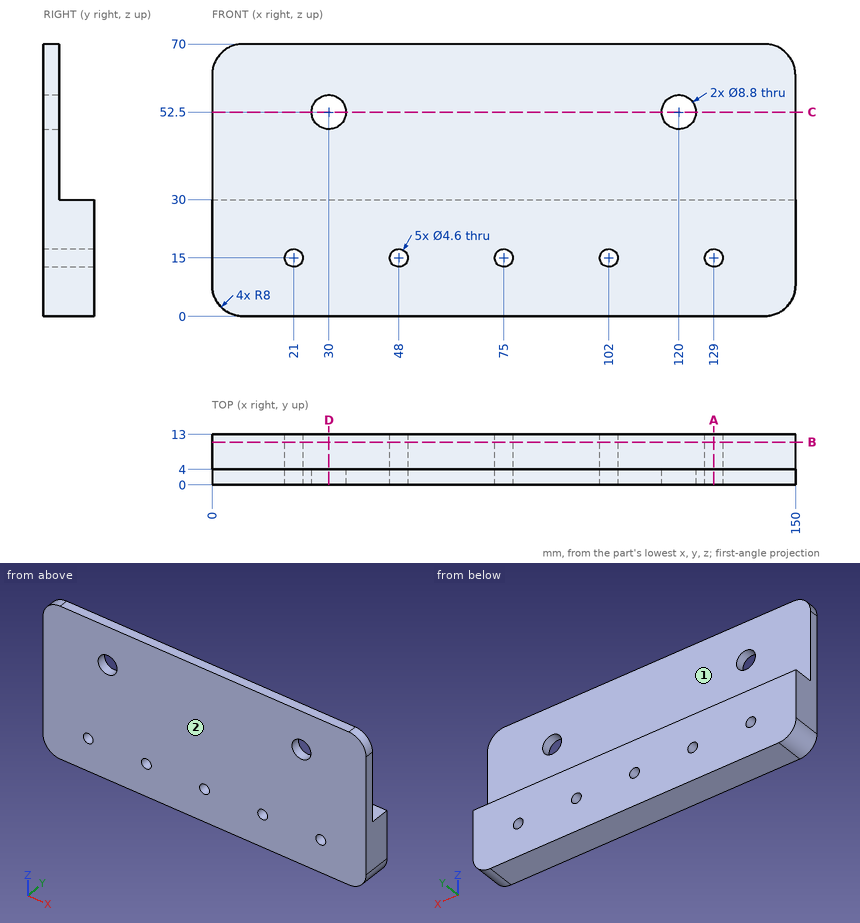
Could you check a few things on this drawing? It's one solid part, dimensions in mm from its lowest x, y, z. A direction names the side the tool comes from. Coordinates: 2 decimals unless noted, no trailing zeros. Write each loop counter-clockwise with the first axis right and the second up, starting at its lowest first coordinate (ties: lowest second). Pieces come first, ordered by that corner, then holes.
1) If we section it at B-B (y = 11): List the corners of the cut face in (x, z) for me.
Filled in:
outline: (0, 8) arc R8 ccw to (8, 0) - (142, 0) arc R8 ccw to (150, 8) - (150, 30) - (0, 30) - close; hole circle Ø4.6 at (21, 15); hole circle Ø4.6 at (48, 15); hole circle Ø4.6 at (75, 15); hole circle Ø4.6 at (102, 15); hole circle Ø4.6 at (129, 15)
2) If I drill on line 1 (X direction, y = 2.5, z = 15); line 2 (Z direction, x = 21, y = 4.75); line 3 (Z direction, x = 30, y = 2.9), over which ranges is the centre line in solid material (lowest first)?
Filled in:
line 1: x = 0 to 18.7, 23.3 to 45.7, 50.3 to 72.7, 77.3 to 99.7, 104.3 to 126.7, 131.3 to 150
line 2: z = 0 to 12.7, 17.3 to 30
line 3: z = 0 to 48.1, 56.9 to 70
3) Which directions (+Z, -Z, +X, -X, +Y, -Y) give clear straight access to the entire face, cutting with the end or side of a thin tool? Please do the marked faces 1 and 2.
Filled in:
face 1: +Z, +X, -X, +Y
face 2: +Z, -Z, +X, -X, -Y
4) If we section it at C-C (z = 52.5): List the corners of the cut face in (x, y) for me.
Filled in:
outline: (0, 0) - (25.6, 0) - (25.6, 4) - (0, 4) - close; (34.4, 0) - (115.6, 0) - (115.6, 4) - (34.4, 4) - close; (124.4, 0) - (150, 0) - (150, 4) - (124.4, 4) - close
5) I'm going to push flat-ended pins straight in: pin 1 (12 mm diameter, centred on x = 50, z = 44.5, fed in from +Y); pin 2 (4.5 mm diameter, centred on x = 65.5, y = 10.5, fed in from +Z). Where does each tip first touch, or does it pass through?
Filled in:
pin 1: stops at y = 4
pin 2: stops at z = 30
6) If we section it at D-D (x = 30): List the corners of the cut face in (y, z) for me, plus the area to 3 significant figures.
Filled in:
outline: (0, 0) - (13, 0) - (13, 30) - (4, 30) - (4, 48.1) - (0, 48.1) - close; (0, 56.9) - (4, 56.9) - (4, 70) - (0, 70) - close
area: 515 mm2
7) If we section it at A-A (x = 129): List the corners of the cut face in (y, z) for me.
Filled in:
outline: (0, 0) - (13, 0) - (13, 12.7) - (0, 12.7) - close; (0, 17.3) - (13, 17.3) - (13, 30) - (4, 30) - (4, 70) - (0, 70) - close
